The model under review builds one solid part; all positions refer to its coordinate system, in mm. A direction names the side the tool comes from. Coordinates: 2 decimals unless noted, no trailing zeros. Order: outer loops, then holes, each group sorted by start corner. A loop starts at its lowest first (then second) coordinate and runs counter-clockwise, first axis right, second up. Notation, with made-up numbers: M 1.5,51.5 L 44.5,51.5 A19 ccw 44.5,86.5 Z; hole C 38,80.5 d2. An arc over 180 degrees is marked long. Answer in a Markdown table with one row per item.
Autodesk Fusion 360 part; units mm, degrees
sketch "Sketch1" plane through (0, 0, 0) normal (0, 1, 0) x (1, 0, 0)
  line L0 (0, 0) -> (40, 0)
  line L1 (40, 0) -> (40, 20)
  line L2 (40, 20) -> (0, 20)
  line L3 (0, 20) -> (0, 0)
  circle A0 centre (8, 10) radius 2.05
  circle A1 centre (20, 10) radius 2.05
  circle A2 centre (32, 10) radius 2.05
  circle A3 centre (8, 10) radius 2.8 construction
  circle A4 centre (32, 10) radius 2.8 construction
  line L4 (5.2, 8.3834) -> (8, 6.7668)
  line L5 (8, 6.7668) -> (10.8, 8.3834)
  line L6 (10.8, 8.3834) -> (10.8, 11.6166)
  line L7 (10.8, 11.6166) -> (8, 13.2332) construction
  line L8 (8, 13.2332) -> (5.2, 11.6166) construction
  line L9 (5.2, 11.6166) -> (5.2, 8.3834)
  line L10 (29.2, 8.3834) -> (32, 6.7668)
  line L11 (32, 6.7668) -> (34.8, 8.3834)
  line L12 (34.8, 8.3834) -> (34.8, 11.6166)
  line L13 (34.8, 11.6166) -> (32, 13.2332) construction
  line L14 (32, 13.2332) -> (29.2, 11.6166) construction
  line L15 (29.2, 11.6166) -> (29.2, 8.3834)
  line L16 (10.8, 11.6166) -> (10.8, 20)
  line L17 (5.2, 11.6166) -> (5.2, 20)
  line L18 (34.8, 11.6166) -> (34.8, 20)
  line L19 (29.2, 11.6166) -> (29.2, 20)
  circle A5 centre (20, 10) radius 1.45
  circle A6 centre (32, 10) radius 1.45
  circle A7 centre (8, 10) radius 1.45
  line L20 (17.2, 8.3834) -> (20, 6.7668)
  line L21 (20, 6.7668) -> (22.8, 8.3834)
  line L22 (22.8, 8.3834) -> (22.8, 11.6166)
  line L23 (22.8, 11.6166) -> (20, 13.2332) construction
  line L24 (20, 13.2332) -> (17.2, 11.6166) construction
  line L25 (17.2, 11.6166) -> (17.2, 8.3834)
  line L26 (17.2, 11.6166) -> (17.2, 20)
  line L27 (22.8, 11.6166) -> (22.8, 20)
  point P0 (8, 10)
  point P1 (32, 10)
  point P2 (20, 10)
  dimension "ClampWidth" = 20
  dimension "ClampLength" = 40
  dimension "MagnetHoleDia" = 4.1
  dimension "d7" = 10
  dimension "d11" = 8
  dimension "d14" = 24
  dimension "d15" = 0
  dimension "NutCircum" = 5.6
  dimension "d17" = 10
  dimension "d19" = 5.6
  dimension "d20" = 8
  dimension "d21" = 10
  dimension "d22" = 2.9
  dimension "ScrewDia" = 2.9
  dimension "d24" = 2.9
extrude "Extrude1" add sketch "Sketch1" along normal blind 20 contours L0 L1 L2 L3 L4 L5 L6 L9 L10 L11 L12 L15 L16 L17 L18 L19 L20 L21 L22 L25 L26 L27 | L2 L4 L5 L6 L9 L16 L17 | L2 L10 L11 L12 L15 L18 L19 | L2 L20 L21 L22 L25 L26 L27 | A0 | A1 | A2 | A5 | A6 | A7
extrude "Extrude2" cut sketch "Sketch1" along normal blind 2.2 contours A0 | A1 | A2 | A5 | A6 | A7
extrude "Extrude3" cut sketch "Sketch1" along normal blind 20 contours A5 | A6 | A7
extrude "Extrude4" cut sketch "Sketch1" against normal blind 2.6 from surface at 15 contours L2 L4 L5 L6 L9 L16 L17 | L2 L10 L11 L12 L15 L18 L19 | L2 L20 L21 L22 L25 L26 L27 | A0 | A1 | A2
fillet "Fillet1" radius 3 4 edges at (40, 10, -20) (40, 10, 0) (0, 10, 0) (0, 10, -20)
chamfer "Chamfer1" distance 3 angle 45 8 edges at (20, 20, -20) (40, 20, -10) (20, 20, 0) (0, 20, -10) (0, 0, -10) (20, 0, -20) (20, 0, 0) (40, 0, -10)
equation "d7 = ClampWidth / 2"
equation "d11 = ClampLength / 5"
equation "d14 = ClampLength * 3 / 5"
equation "d17 = ClampWidth / 2"
equation "d19 = NutCircum"
equation "d20 = ClampLength / 5"
equation "d21 = ClampWidth / 2"
equation "d22 = ScrewDia"
equation "d24 = ScrewDia"
equation "d29 = TotalHeight"
equation "NutTopOffset = 5 mm"
equation "NutWidth = 2.6 mm"
equation "d33 = TotalHeight - NutTopOffset"
(1) Take a section at C-C (x = 25.5). Write out the cut boundary in (y, z).
Report:
| item | result |
|---|---|
| outline | M 0,-17 L 3,-20 L 17,-20 L 20,-17 L 20,-3 L 17,0 L 3,0 L 0,-3 Z |
(2) Take a section at D-D (z = -10). State how many separate pieces and enclosed holes the cut face has, then the cut area to 3 significant figures.
Report:
| item | result |
|---|---|
| separate pieces | 4 |
| enclosed holes | 0 |
| area | 579 mm^2 |
(3) Insertion check: P1, Ø2.5, axis at x = 8, z = -10, coming from the +Y side; P2, Ø1.2, axis at x = 33, z = -9.5, coming from the -Y side. Each pin has a flat end and moves straight along its axis. Give the tip position at first contact, or say it passes through.
Report:
| item | result |
|---|---|
| P1 | through |
| P2 | y = 2.2 |
(4) Take a section at B-B (z = -13.75). Write out the cut boundary in (x, y).
Report:
| item | result |
|---|---|
| outline | M 0,3 L 3,0 L 37,0 L 40,3 L 40,17 L 37,20 L 3,20 L 0,17 Z; hole M 5.2,12.4 L 10.8,12.4 L 10.8,15 L 5.2,15 Z; hole M 17.2,12.4 L 22.8,12.4 L 22.8,15 L 17.2,15 Z; hole M 29.2,12.4 L 34.8,12.4 L 34.8,15 L 29.2,15 Z |
(5) To check wall thickness, follow line 1 (X direction, y = 5.25, z = -10); line 2 (X direction, y = 14.75, z = -9.5); line 3 (Y direction, x = 30, z = -11.5). State the ranges of each line that lie inside material, in increasing order. Write a range as [from, to].
Report:
| item | result |
|---|---|
| line 1 | [0, 6.55], [9.45, 18.55], [21.45, 30.55], [33.45, 40] |
| line 2 | [0, 5.2], [10.8, 17.2], [22.8, 29.2], [34.8, 40] |
| line 3 | [0, 12.4], [15, 20] |
(6) Machinability: for faces 1 (the flat face through (2, 1, -10)), 2 (the flat face through (10.8, 14, -14)), 3 (the flat face through (9.34, 2.2, -9.12)), which of the approach directions +Z, -Z, +X, -X, +Y, -Y give a long, thin tool a straight path to every point of the face, cutting with its end or side? Answer none if there is none.
Report:
| item | result |
|---|---|
| face 1 | +Z, -Z, -X, -Y |
| face 2 | -Z |
| face 3 | -Y |
(7) The part is to be moulded in two halves that separate along Y. For faces 4 (the flat face through (34.8, 14, -14)), 5 (the flat face through (29.2, 14, -14)), 6 (the conical face through (38.09, 1.52, -18.06)), 7 (the flat face through (40, 10, -10)), say which applies: +Y half, -Y half, draft (parallel to the pull), parting line (faces both ways), or undercut.
Report:
| item | result |
|---|---|
| face 4 | undercut |
| face 5 | undercut |
| face 6 | -Y half |
| face 7 | draft |
(8) Take a section at A-A (y = 9.5). Write out the cut boundary in (x, z), then the cut area to 3 significant figures.
Report:
| item | result |
|---|---|
| outline | M 0,-17 A3 ccw 3,-20 L 37,-20 A3 ccw 40,-17 L 40,-3 A3 ccw 37,0 L 3,0 A3 ccw 0,-3 Z; hole C 8,-10 d2.9; hole C 20,-10 d2.9; hole C 32,-10 d2.9 |
| area | 772 mm^2 |
